```python
from build123d import *

# Parameters (mm, degrees)
SKETCH1_W               = 5.6
SKETCH1_H               = 40
BOSS_EXTRUDE1_DEPTH     = 4
SKETCH2_W               = 5.6
SKETCH2_H               = 2
BOSS_EXTRUDE2_DEPTH     = 4
SKETCH4_W               = 4
SKETCH4_H               = 4.2
BOSS_EXTRUDE3_DEPTH     = 1.8
MIRROR2_COPY_1_SKETCH_W = 4
MIRROR2_COPY_1_SKETCH_H = 4.2
MIRROR2_COPY_1_DEPTH    = 1.8
SKETCH8_W               = 4
SKETCH8_H               = 4.2
BOSS_EXTRUDE4_DEPTH     = 8
SKETCH9_W               = 17.2
SKETCH9_H               = 2.1
BOSS_EXTRUDE5_DEPTH     = 4


with BuildPart() as part:
    # Sketch1 → Boss-Extrude1 (new body)
    with BuildSketch(Plane.XY):
        Rectangle(SKETCH1_W, SKETCH1_H)
    extrude(amount=BOSS_EXTRUDE1_DEPTH)

    # Sketch2 → Boss-Extrude2 (add)
    with BuildSketch(Plane.XY.offset(4)):
        with Locations((0, -19)):
            Rectangle(SKETCH2_W, SKETCH2_H)
    extrude(amount=BOSS_EXTRUDE2_DEPTH)

    # Sketch4 → Boss-Extrude3 (add)
    with BuildSketch(Plane.ZY.offset(2.8)):
        with Locations((2, 9.6)):
            Rectangle(SKETCH4_W, SKETCH4_H)
    boss_extrude3 = extrude(amount=BOSS_EXTRUDE3_DEPTH)

    # Mirror1: Boss-Extrude3 across plane
    add(boss_extrude3.mirror(Plane.ZY))

    # Mirror2: Boss-Extrude3 across plane
    add(boss_extrude3.mirror(Plane(origin=(0, 1.1, 0), x_dir=(0, 0, 1), z_dir=(0, -1, 0))))

    # Mirror2 copy 1 sketch → Mirror2 copy 1 (add)
    with BuildSketch(Plane(origin=(2.8, 2.2, 0), x_dir=(0, 0, 1), z_dir=(1, 0, 0))):
        with Locations((2, 9.6)):
            Rectangle(MIRROR2_COPY_1_SKETCH_W, MIRROR2_COPY_1_SKETCH_H)
    extrude(amount=MIRROR2_COPY_1_DEPTH)

    # Sketch8 → Boss-Extrude4 (add)
    with BuildSketch(Plane.ZY.offset(4.6)):
        with Locations((2, 9.6)):
            Rectangle(SKETCH8_W, SKETCH8_H)
        with Locations((2, -7.4)):
            Rectangle(SKETCH8_W, SKETCH8_H)
    extrude(amount=BOSS_EXTRUDE4_DEPTH)

    # Sketch9 → Boss-Extrude5 (add)
    with BuildSketch(Plane.XY.offset(4)):
        with Locations((-4, 10.65)):
            Rectangle(SKETCH9_W, SKETCH9_H)
    extrude(amount=BOSS_EXTRUDE5_DEPTH)


solid = part.part
```
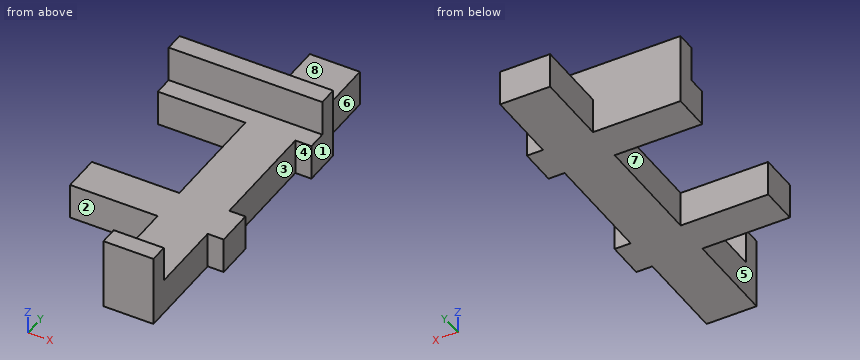
The model under review builds one solid part; all positions refer to its coordinate system, in mm. Face numbers are marked on the shaded views. A direction names the side the tool comes from. Give positions to 0.01 mm unless a question says otherwise; leave off trailing zeros. Write each loop counter-clockwise with the first axis right and the second up, starting at its lowest first coordinate (ties: lowest second). Pieces come first, ordered by that corner, then holes. Notation, with made-up numbers: (-27.5, 52) - (-16.5, 52) arc R34 cw to (-16.5, 85) - close; hole circle Ø4 at (47, 16.5). An arc over 180 degrees is marked (long way). Answer in a Markdown table with one row per item. Add a question column.
1. We need section B-B on x = -4.5. Write out the cut boundary in (y, z).
2. Draft analysis for pull direction Y (two halves, no side actions). For the marked faces 1, 2 and 3, state which applies: +Y half, -Y half, draft (parallel to the pull), parting line (faces both ways), or undercut.
3. Insertion check: P1, Ø2.5, axis at y = -17, z = 4.5, coming from the +X side; P2, Ø3, axis at x = -0.5, y = 17.5, coming from the +Z side; P3, Ø0.9, axis at x = 3.5, z = 1.5, coming from the -Y side; P4, Ø2, axis at x = -1, y = -1, coming from the -Z side. Each pin has a flat end and moves straight along its axis. Give the tip position at first contact, or say it passes through.
4. We need section D-D on z = 3. Write out the cut boundary in (x, y).
5. Wall thickness on line 1 along Y through (x, z) = (4.25, 2); line 2 along Y through (x, z) = (-2.5, 4.5); line 3 along X through (y, z) = (-17, 2.25): over which ranges is each line inside the solid? List them lowest first. Write a range as [from, to].
6. We need section A-A on z = 4.75. Write out the cut boundary in (x, y), then the cut area to 3 significant figures.
7. Tool access review of the marked faces 4, 5, 6, 7 and 8: name each direction out of +Z, -Z, +X, -X, +Y, -Y from which nothing blocks a thin tool from reaching the whole face with its end or side.
8. We need section C-C on x = 1.5. Write out the cut boundary in (y, z), then the cut area to 3 significant figures.
Ans:
| question | item | result |
|---|---|---|
| 1 | outline | (-9.5, 0) - (-5.3, 0) - (-5.3, 4) - (-9.5, 4) - close; (7.5, 0) - (11.7, 0) - (11.7, 8) - (9.6, 8) - (9.6, 4) - (7.5, 4) - close |
| 2 | face 1 | draft |
| 2 | face 2 | -Y half |
| 2 | face 3 | undercut |
| 3 | P1 | stops at x = 2.8 |
| 3 | P2 | stops at z = 4 |
| 3 | P3 | stops at y = -9.5 |
| 3 | P4 | stops at z = 0 |
| 4 | outline | (-12.6, -9.5) - (-2.8, -9.5) - (-2.8, -20) - (2.8, -20) - (2.8, -9.5) - (4.6, -9.5) - (4.6, -5.3) - (2.8, -5.3) - (2.8, 7.5) - (4.6, 7.5) - (4.6, 11.7) - (2.8, 11.7) - (2.8, 20) - (-2.8, 20) - (-2.8, 11.7) - (-12.6, 11.7) - (-12.6, 7.5) - (-2.8, 7.5) - (-2.8, -5.3) - (-12.6, -5.3) - close |
| 5 | line 1 | y = [-9.5, -5.3], [7.5, 11.7] |
| 5 | line 2 | y = [-20, -18], [9.6, 11.7] |
| 5 | line 3 | x = [-2.8, 2.8] |
| 6 | outline | (-12.6, 9.6) - (4.6, 9.6) - (4.6, 11.7) - (-12.6, 11.7) - close; (-2.8, -20) - (2.8, -20) - (2.8, -18) - (-2.8, -18) - close |
| 6 | area | 47.3 mm^2 |
| 7 | face 4 | +Z, -Z, +X |
| 7 | face 5 | +Z, -Z, -X, -Y |
| 7 | face 6 | +Z, -Z, +X, +Y |
| 7 | face 7 | +Z, -Z, -X |
| 7 | face 8 | +Z, +X, -X, +Y |
| 8 | outline | (-20, 0) - (20, 0) - (20, 4) - (11.7, 4) - (11.7, 8) - (9.6, 8) - (9.6, 4) - (-18, 4) - (-18, 8) - (-20, 8) - close |
| 8 | area | 176 mm^2 |
